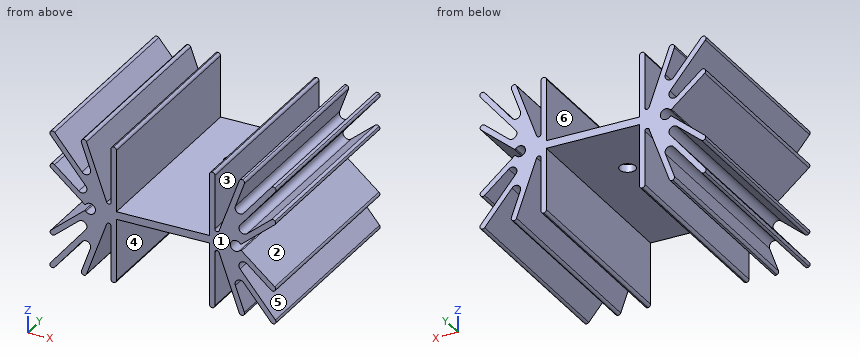
```python
from build123d import *

# Parameters (mm, degrees)
INNER_HALF_DEPTH          = 18
FLANGES_REACH             = 25.885
FLANGES_DIRECTION_2_REACH = 25.885
FILLET1_R                 = 0.5
FILLET1_OF_MIRROR1_R      = 0.5
MIRROR3_START             = -18
MIRROR3_DEPTH             = 36
SKETCH3_R                 = 1
INNER_CIRCLE_DEPTH        = 44.391544118
M3_5X0_6_TAPPED_HOLE1_D   = 2.9
FILLET3_R                 = 0.2
FILLET2_R                 = 0.5


# Read off the part's stored shape, not the designer's step: Mirror3
with BuildPart() as part:
    # Sketch1 → INNER HALF (new, symmetric)
    with BuildSketch(Plane(origin=(0, 0, 0), x_dir=(1, 0, 0), z_dir=(0, 1, 0))):
        Polygon((-8.5, 0.7), (0, 0.7), (0, -0.7), (-8.5, -0.7), (-8.5, -12.5), (-9.5, -12.5), (-9.5, 12.5), (-8.5, 12.5), align=None)
    inner_half = extrude(amount=INNER_HALF_DEPTH, both=True)

    # Mirror2: INNER HALF across plane
    add(inner_half.mirror(Plane(origin=(0, 0, 0), x_dir=(0, 0, 1), z_dir=(1, 0, 0))))

    # FLANGES: up to this face of the body (flat: up to its plane)
    flanges_end = Plane(part.part.faces().sort_by_distance((0, 18, 0))[0])
    # Sketch2 → FLANGES (add, up to the picked face)
    with BuildSketch(Plane(origin=(0, 0, 0), x_dir=(1, 0, 0), z_dir=(0, 1, 0)), mode=Mode.PRIVATE) as flanges_sk1:
        with BuildLine():
            Line((-10.276164759, 2.012372382), (-14.129794052, 12.670018723))
            Line((-14.129794052, 12.670018723), (-15.070205948, 12.329981277))
            Line((-15.070205948, 12.329981277), (-13.253629293, 7.306033701))
            ThreePointArc((-13.253629293, 7.306033701), (-13.652352407, 6.219223699), (-14.791703546, 6.42419951))
            Line((-14.791703546, 6.42419951), (-20.115720252, 12.819889161))
            Line((-20.115720252, 12.819889161), (-20.884279748, 12.180110839))
            Line((-20.884279748, 12.180110839), (-14.108296454, 4.040187803))
            ThreePointArc((-14.108296454, 4.040187803), (-14.164853061, 2.826744492), (-15.378508849, 2.774947314))
            Line((-15.378508849, 2.774947314), (-20.178606195, 6.802707227))
            Line((-20.178606195, 6.802707227), (-20.821393805, 6.036662784))
            Line((-20.821393805, 6.036662784), (-13.627179245, 0))
            Line((-13.627179245, 0), (-9.5, 0))
            Line((-9.5, 0), (-9.5, 2.14838736))
            ThreePointArc((-9.5, 2.14838736), (-9.830956186, 1.754391228), (-10.276164759, 2.012372382))
        make_face()
    flanges_tool1 = split(extrude(flanges_sk1.sketch, amount=FLANGES_REACH, mode=Mode.PRIVATE), bisect_by=flanges_end, keep=Keep.BOTH, mode=Mode.PRIVATE)
    flanges = flanges_tool1.solids().sort_by(Axis((-14.387215, 0, -5.095322), (0, 1, 0)))[0]
    add(flanges)

    # FLANGES direction 2: up to this face of the body (flat: up to its plane)
    flanges_direction_2_end = Plane(part.part.faces().sort_by_distance((0, -18, 0))[0])
    # Sketch2 → FLANGES direction 2 (add, up to the picked face)
    with BuildSketch(Plane(origin=(0, 0, 0), x_dir=(1, 0, 0), z_dir=(0, 1, 0)), mode=Mode.PRIVATE) as flanges_direction_2_sk1:
        with BuildLine():
            Line((-10.276164759, 2.012372382), (-14.129794052, 12.670018723))
            Line((-14.129794052, 12.670018723), (-15.070205948, 12.329981277))
            Line((-15.070205948, 12.329981277), (-13.253629293, 7.306033701))
            ThreePointArc((-13.253629293, 7.306033701), (-13.652352407, 6.219223699), (-14.791703546, 6.42419951))
            Line((-14.791703546, 6.42419951), (-20.115720252, 12.819889161))
            Line((-20.115720252, 12.819889161), (-20.884279748, 12.180110839))
            Line((-20.884279748, 12.180110839), (-14.108296454, 4.040187803))
            ThreePointArc((-14.108296454, 4.040187803), (-14.164853061, 2.826744492), (-15.378508849, 2.774947314))
            Line((-15.378508849, 2.774947314), (-20.178606195, 6.802707227))
            Line((-20.178606195, 6.802707227), (-20.821393805, 6.036662784))
            Line((-20.821393805, 6.036662784), (-13.627179245, 0))
            Line((-13.627179245, 0), (-9.5, 0))
            Line((-9.5, 0), (-9.5, 2.14838736))
            ThreePointArc((-9.5, 2.14838736), (-9.830956186, 1.754391228), (-10.276164759, 2.012372382))
        make_face()
    flanges_direction_2_tool1 = split(extrude(flanges_direction_2_sk1.sketch, amount=-FLANGES_DIRECTION_2_REACH, mode=Mode.PRIVATE), bisect_by=flanges_direction_2_end, keep=Keep.BOTH, mode=Mode.PRIVATE)
    flanges_direction_2 = flanges_direction_2_tool1.solids().sort_by(Axis((-14.387215, 0, -5.095322), (0, -1, 0)))[0]
    add(flanges_direction_2)

    # Fillet1
    fillet1_edges = [part.edges().sort_by_distance(p)[0] for p in [
        (-20.821393805, 0, -6.036662784),
        (-20.178606195, 0, -6.802707227),
        (-20.115720252, 0, -12.819889161),
        (-20.884279748, 0, -12.180110839),
        (-14.129794052, 0, -12.670018723),
        (-15.070205948, 0, -12.329981277),
    ]]
    fillet(fillet1_edges, radius=FILLET1_R - 0.0001)  # a hair under: the kernel refuses the full size

    # Mirror1: FLANGES, FLANGES direction 2 across plane
    add(flanges.mirror(Plane.XY))
    add(flanges_direction_2.mirror(Plane.XY))

    # Fillet1 of Mirror1
    fillet1_of_mirror1_edges = [part.edges().sort_by_distance(p)[0] for p in [
        (-20.821393805, 0, 6.036662784),
        (-20.178606195, 0, 6.802707227),
        (-20.115720252, 0, 12.819889161),
        (-20.884279748, 0, 12.180110839),
        (-14.129794052, 0, 12.670018723),
        (-15.070205948, 0, 12.329981277),
    ]]
    fillet(fillet1_of_mirror1_edges, radius=FILLET1_OF_MIRROR1_R - 0.0001)  # a hair under: the kernel refuses the full size

    # Mirror3 outline → Mirror3 (add)
    with BuildSketch(Plane(origin=(0, 0, 0), x_dir=(1, 0, 0), z_dir=(0, 1, 0)).offset(MIRROR3_START)):
        with BuildLine():
            ThreePointArc((14.6, 12.5), (14.217716854, 12.482501258), (13.959775329, 12.199812774))
            Line((13.959775329, 12.199812774), (10.276164759, 2.012372382))
            ThreePointArc((10.276164759, 2.012372382), (9.830956186, 1.754391228), (9.5, 2.14838736))
            Line((9.5, 2.14838736), (9.5, -2.14838736))
            ThreePointArc((9.5, -2.14838736), (9.830956186, -1.754391228), (10.276164759, -2.012372382))
            Line((10.276164759, -2.012372382), (13.959775329, -12.199812774))
            ThreePointArc((13.959775329, -12.199812774), (14.217716854, -12.482501258), (14.6, -12.5))
            ThreePointArc((14.6, -12.5), (14.882688484, -12.242058475), (14.900187226, -11.859775329))
            Line((14.900187226, -11.859775329), (13.253629293, -7.306033701))
            ThreePointArc((13.253629293, -7.306033701), (13.652352407, -6.219223699), (14.791703546, -6.42419951))
            Line((14.791703546, -6.42419951), (19.795831091, -12.435609413))
            ThreePointArc((19.795831091, -12.435609413), (20.134579818, -12.613642863), (20.5, -12.5))
            ThreePointArc((20.5, -12.5), (20.67803345, -12.161251273), (20.564390587, -11.795831091))
            Line((20.564390587, -11.795831091), (14.108296454, -4.040187803))
            ThreePointArc((14.108296454, -4.040187803), (14.164853061, -2.826744492), (15.378508849, -2.774947314))
            Line((15.378508849, -2.774947314), (19.795583974, -6.481313422))
            ThreePointArc((19.795583974, -6.481313422), (20.16055565, -6.59638855), (20.5, -6.419685006))
            ThreePointArc((20.5, -6.419685006), (20.615075127, -6.054713329), (20.438371583, -5.715268979))
            Line((20.438371583, -5.715268979), (13.627179245, 0))
            Line((13.627179245, 0), (20.438371583, 5.715268979))
            ThreePointArc((20.438371583, 5.715268979), (20.615075127, 6.054713329), (20.5, 6.419685006))
            ThreePointArc((20.5, 6.419685006), (20.16055565, 6.59638855), (19.795583974, 6.481313422))
            Line((19.795583974, 6.481313422), (15.378508849, 2.774947314))
            ThreePointArc((15.378508849, 2.774947314), (14.164853061, 2.826744492), (14.108296454, 4.040187803))
            Line((14.108296454, 4.040187803), (20.564390587, 11.795831091))
            ThreePointArc((20.564390587, 11.795831091), (20.67803345, 12.161251273), (20.5, 12.5))
            ThreePointArc((20.5, 12.5), (20.134579818, 12.613642863), (19.795831091, 12.435609413))
            Line((19.795831091, 12.435609413), (14.791703546, 6.42419951))
            ThreePointArc((14.791703546, 6.42419951), (13.652352407, 6.219223699), (13.253629293, 7.306033701))
            Line((13.253629293, 7.306033701), (14.900187226, 11.859775329))
            ThreePointArc((14.900187226, 11.859775329), (14.882688484, 12.242058475), (14.6, 12.5))
        make_face()
    extrude(amount=MIRROR3_DEPTH)

    # Sketch3 → INNER CIRCLE (cut, symmetric)
    with BuildSketch(Plane(origin=(0, 18, 0), x_dir=(1, 0, 0), z_dir=(0, 1, 0))):
        with Locations((-13.327179245, 0)):
            Circle(SKETCH3_R)
    inner_circle = extrude(amount=INNER_CIRCLE_DEPTH, both=True, mode=Mode.SUBTRACT)

    # Mirror6: INNER CIRCLE across plane
    add(inner_circle.mirror(Plane(origin=(0, 0, 0), x_dir=(0, 0, 1), z_dir=(1, 0, 0))), mode=Mode.SUBTRACT)

    # M3.5x0.6 Tapped Hole1 (through all)
    with Locations(Plane.XY.offset(0.7)):
        with Locations((0, 6)):
            Hole(M3_5X0_6_TAPPED_HOLE1_D / 2)

    # Fillet3
    fillet3_edges = [part.edges().sort_by_distance(p)[0] for p in [
        (-14.202798531, 0, 0.483001931),
        (-14.202798531, 0, -0.483001931),
        (14.202798531, 0, 0.483001931),
        (14.202798531, 0, -0.483001931),
    ]]
    fillet(fillet3_edges, radius=FILLET3_R)

    # Fillet2
    fillet2_edges = [part.edges().sort_by_distance(p)[0] for p in [
        (-8.5, 0, 12.5),
        (-9.5, 0, 12.5),
        (-8.5, 0, -12.5),
        (-9.5, 0, -12.5),
        (9.5, 0, 12.5),
        (8.5, 0, 12.5),
        (9.5, 0, -12.5),
        (8.5, 0, -12.5),
    ]]
    fillet(fillet2_edges, radius=FILLET2_R - 0.0001)  # a hair under: the kernel refuses the full size


solid = part.part
```
The model under review builds one solid part; all positions refer to its coordinate system, in mm. Face numbers are marked on the shaded views. A direction names the side the tool comes from. Round coordinates to 2 decimals unless told otherwise and drop trailing zeros. Order: outer loops, then holes, each group sorted by start corner. A loop starts at its lowest first (then second) coordinate and runs counter-clockwise, first axis right, second up. Notation, with made-up numbers: (74.25, 32.25) -> (78.25, 32.25) arc R17 cw to (78.25, 60.25) -> close; hole circle Ø9 at (-9.75, 3). An arc over 180 degrees is marked (long way). One line per item, written item: value. Start each with the question number.
Q1. Take a section at B-B (z = -11). Write out the cut boundary in (x, y).
Q2. Mouldability with a two-part tool opening along X and no side actions: class the marked faces 1, 2 and 3 as released by +X, released by -X, zero draft, split by the parting line, or undercut.
Q3. Machinability: for the marked faces 4, 5 and 6, which of the approach directions +Z, -Z, +X, -X, +Y, -Y give a long, thin tool a straight path to every point of the face, cutting with its end or side? Answer none if there is none.
Q4. Take a section at A-A (x = 0). Write out the cut boundary in (y, z), and give its area (3 significant figures).
Q5. Clearance check with flat-ended pins moving along their axes: pin 1 Ø5 at (y, z) = (-12, -1) entering from +X; pin 2 Ø1.5 at (y, z) = (5, 5.5) entering from +X; pin 3 Ø3.5 at (y, z) = (8, 5) entering from -X. State where each tip first meets the part, or that it passes through.
Q6. Take a section at D-D (x = -5). Write out the cut boundary in (y, z), and give its area (3 significant figures).
Q7. Take a section at C-C (z = 0). Write out the cut boundary in (x, y), and give its area (3 significant figures).
Q8. Wall thickness on line 1 (Z direction, x = 19.5, y = -8); line 2 (Y direction, x = 0, z = 0); line 3 (X direction, y = -0.5, z = 2.75): over which ranges is each line inside the solid? List them lowest first.
Reported:
1. outline: (-19.9, -18) -> (-18.6, -18) -> (-18.6, 18) -> (-19.9, 18) -> close; (-14.59, -18) -> (-13.53, -18) -> (-13.53, 18) -> (-14.59, 18) -> close; (-9.5, -18) -> (-8.5, -18) -> (-8.5, 18) -> (-9.5, 18) -> close; (8.5, -18) -> (9.5, -18) -> (9.5, 18) -> (8.5, 18) -> close; (13.53, -18) -> (14.59, -18) -> (14.59, 18) -> (13.53, 18) -> close; (18.6, -18) -> (19.9, -18) -> (19.9, 18) -> (18.6, 18) -> close
2. face 1: zero draft
2. face 2: released by +X
2. face 3: undercut
3. face 4: -Z, +Y, -Y
3. face 5: +Y, -Y
3. face 6: +Z, +Y, -Y
4. outline: (-18, -0.7) -> (4.55, -0.7) -> (4.55, 0.7) -> (-18, 0.7) -> close; (7.45, -0.7) -> (18, -0.7) -> (18, 0.7) -> (7.45, 0.7) -> close
4. area: 46.3 mm2
5. pin 1: stops at x = 17.8
5. pin 2: stops at x = 20.62
5. pin 3: stops at x = -20.62
6. outline: (-18, -0.7) -> (18, -0.7) -> (18, 0.7) -> (-18, 0.7) -> close
6. area: 50.4 mm2
7. outline: (-12.33, -18) -> (12.33, -18) -> (12.33, 18) -> (-12.33, 18) -> close; hole circle Ø2.9 at (0, 6)
7. area: 881 mm2
8. line 1: z = -12.08 to -10.52, -6.23 to -4.93, 4.93 to 6.23, 10.52 to 12.08
8. line 2: y = -18 to 4.55, 7.45 to 18
8. line 3: x = -16.9 to -15.35, -14.25 to -10.54, -9.5 to -8.5, 8.5 to 9.5, 10.54 to 14.25, 15.35 to 16.9
